from build123d import *

# Parameters (mm, degrees)
SKETCH_R     = 10
PAD_DEPTH    = 40
PAD001_DEPTH = 10
FILLET_R     = 1


with BuildPart() as part:
    # Sketch → Pad (new body)
    with BuildSketch(Plane.XY):
        Circle(SKETCH_R)
    extrude(amount=PAD_DEPTH)

    # Sketch001 → Pad001 (join)
    with BuildSketch(Plane.XY):
        Polygon((15, 0), (7.5, 12.990381), (-7.5, 12.990381), (-15, 0), (-7.5, -12.990381), (7.5, -12.990381), align=None)
    extrude(amount=PAD001_DEPTH)

    # Fillet
    fillet_edges = [part.edges().sort_by_distance(p)[0] for p in [
        (-7.5, -12.990381, 5),
        (7.5, -12.990381, 5),
        (0, -12.990381, 0),
        (0, -12.990381, 10),
        (15, 0, 5),
        (11.25, -6.495191, 0),
        (11.25, -6.495191, 10),
        (11.25, 6.495191, 10),
        (0, 12.990381, 10),
        (-11.25, 6.495191, 10),
        (-11.25, -6.495191, 10),
        (-10, 0, 10),
        (-15, 0, 5),
        (-11.25, -6.495191, 0),
        (-7.5, 12.990381, 5),
        (-11.25, 6.495191, 0),
        (11.25, 6.495191, 0),
        (0, 12.990381, 0),
        (7.5, 12.990381, 5),
    ]]
    fillet(fillet_edges, radius=FILLET_R)


solid = part.part
For this review, take the finished solid that the model builds, in its own axes (mm). A direction names the side the tool comes from. Coordinates: 2 decimals unless noted, no trailing zeros. Order: outer loops, then holes, each group sorted by start corner. A loop starts at its lowest first (then second) coordinate and runs counter-clockwise, first axis right, second up. Notation, with made-up numbers: (63, -16.5) - (92, -16.5) arc R18 ccw to (92, -10.5) - close; hole circle Ø6 at (68.5, 78.5). An arc over 180 degrees is marked (long way). Answer as CSV lines item,"result". Start each with the question number.
1) Add section B-B (z = 15). State the section outline as (x, y) points.
2) Insertion check: P1, Ø3, axis at y = 1, z = 21.5, coming from the -X side; P2, Ø10, axis at x = -5.5, z = 25, coming from the -Y side; P3, Ø1, axis at y = -8.5, z = 16.5, coming from the +X side. Each pin has a flat end and moves straight along its axis. Give the tip position at first contact, or say it passes through.
3) To check wall thickness, follow line 1 along Z through (x, y) = (-5.75, 11.5); line 2 along X through (y, z) = (-1.5, 12); line 3 along X through (y, z) = (-7.25, 26.5). State the ranges of each line that lie inside material, in increasing order. Write a range as [from, to].
4) Machinability: for faces 1 (the flat face through (11.2, -6.58, 4.94)), 2 (the cylindrical face through (-2.17, -9.76, 25.3)), which of the approach directions +Z, -Z, +X, -X, +Y, -Y give a long, thin tool a straight path to every point of the face, cutting with its end or side? Answer none if there is none.
5) Add section A-A (x = 0). State the section outline as (y, z) points.
Result:
1,outline,"circle Ø20 at (0, 0)"
2,P1,"x = -10"
2,P2,"y = -9.99"
2,P3,"x = 6"
3,line 1,"[0, 10]"
3,line 2,"[-9.89, 9.89]"
3,line 3,"[-6.89, 6.89]"
4,face 1,"+Z, -Z, +X, -Y"
4,face 2,"+Z"
5,outline,"(-12.99, 1) arc R1 ccw to (-11.99, 0) - (11.99, 0) arc R1 ccw to (12.99, 1) - (12.99, 9) arc R1 ccw to (11.99, 10) - (11, 10) arc R1 cw to (10, 11) - (10, 40) - (-10, 40) - (-10, 11) arc R1 cw to (-11, 10) - (-11.99, 10) arc R1 ccw to (-12.99, 9) - close"
